Read the model definition and answer for the solid it produces. Units are mm, in the model's axes. Face numbers are marked on the shaded views. A direction names the side the tool comes from. Give positions to 0.01 mm unless a question says otherwise; leave off trailing zeros. Order: outer loops, then holes, each group sorted by start corner. A loop starts at its lowest first (then second) coordinate and runs counter-clockwise, first axis right, second up. Notation, with made-up numbers: (64.25, 17) -> (86.25, 17) arc R13 cw to (86.25, 31) -> close; hole circle Ø9 at (10.25, 18.5). An arc over 180 degrees is marked (long way). Answer as CSV lines item,"result". Start each with the question number.
1) Find section A-A (x = -8.5). Determine the outline of the cut face in (y, z), and give its area (3 significant figures).
2) Find section B-B (z = 61). Determine the outline of the cut face in (x, y).
3) The mould has two halves that part along X. Classify the marked faces 6, 7 and 8: +X half, -X half, draft (parallel to the pull), parting line (faces both ways), or undercut.
4) For the marked faces 1, 2, 3, 4 and 5, determine the directions among +Z, -Z, +X, -X, +Y, -Y from which every point of the face is accessible in a straight line to the end or side of a thin tool.
5) Straight lines are drawn through the part: L1, parallel to Z at x = -5, y = -15.5; L2, parallel to Z at x = -21, y = -19.25; L3, parallel to X at y = -24.75, z = 2. For each, find the intervals that lie inside material, in ascending order. Write a range as from..to.
6) Flat-ended cylindrical pins translate along their axes: pin 1 Ø8 at (x, y) = (19, -19.5) entering from +Z; pin 2 Ø12 at (y, z) = (-16, 94.5) entering from -X; pin 3 Ø1 at (y, z) = (-5, 99) entering from +X. Find the tip coordinate at first contact, or state that the pin passes through.
7) Find section C-C (y = -15). Determine the outline of the cut face in (x, z), and give its area (3 significant figures).
8) Find section D-D (x = -23.5). Determine the outline of the cut face in (y, z).
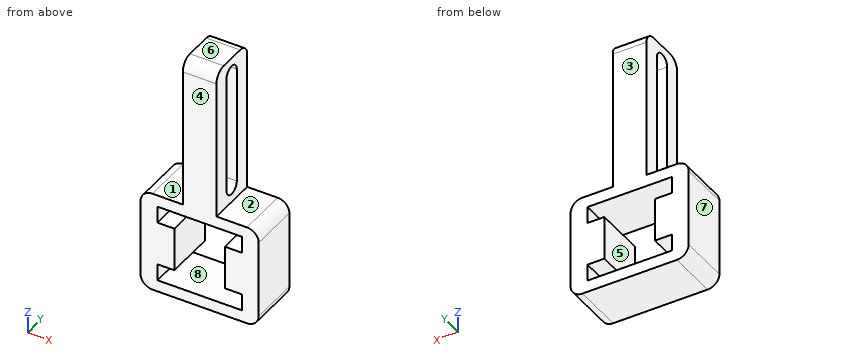
```python
from build123d import *

# Parameters (mm, degrees)
F0_W     = 20
F0_H     = 90
F1_DEPTH = 30
F3_DEPTH = 82
F5_R     = 7
F7_DEPTH = 40.5


with BuildPart() as f1:
    # F0 (on Front) → F1 (new body)
    with BuildSketch(Plane.XZ):
        with BuildLine():
            Line((-28, -30), (28, -30))
            ThreePointArc((28, -30), (32.949747, -27.949747), (35, -23))
            Line((35, -23), (35, 23))
            ThreePointArc((35, 23), (32.949747, 27.949747), (28, 30))
            Line((28, 30), (10, 30))
            Line((10, 30), (-10, 30))
            Line((-10, 30), (-28, 30))
            ThreePointArc((-28, 30), (-32.949747, 27.949747), (-35, 23))
            Line((-35, 23), (-35, -23))
            ThreePointArc((-35, -23), (-32.949747, -27.949747), (-28, -30))
        make_face()
        with Locations((0, 75)):
            Rectangle(F0_W, F0_H)
    extrude(amount=F1_DEPTH)


with BuildPart() as f3:
    # F2 (on face) → F3 (new body, symmetric)
    with BuildSketch(Plane.XZ.offset(30)):
        Polygon((25, 23.023667), (0, 23.023667), (-25, 23.023667), (-25, 13.023667), (-15, 13.023667), (-15, 0.299923), (-15, -0.299923), (-15, -13.023667), (-25, -13.023667), (-25, -23.023667), (0, -23.023667), (25, -23.023667), (25, -13.023667), (15, -13.023667), (15, -0.299923), (15, 0.299923), (15, 13.023667), (25, 13.023667), align=None)
    extrude(amount=F3_DEPTH, both=True)


with BuildPart() as f1_1:
    add(f1.part)

    # F4: cut F3
    add(f3.part, mode=Mode.SUBTRACT)

    # F5
    f5_edges = [f1_1.edges().sort_by_distance(p)[0] for p in [
        (0, -30, 120),
        (0, 0, 120),
    ]]
    fillet(f5_edges, radius=F5_R)


with BuildPart() as f7:
    # F6 (on face) → F7 (new body)
    with BuildSketch(Plane.YZ.offset(10)):
        with BuildLine():
            ThreePointArc((-10.195938, 110), (-15.195938, 115), (-20.195938, 110))
            Line((-20.195938, 110), (-20.195938, 40))
            ThreePointArc((-20.195938, 40), (-15.195938, 35), (-10.195938, 40))
            Line((-10.195938, 40), (-10.195938, 110))
        make_face()
    extrude(amount=-F7_DEPTH)


with BuildPart() as f1_2:
    add(f1_1.part)

    # F8: cut F7
    add(f7.part, mode=Mode.SUBTRACT)


solid = f1_2.part
```
Findings below:
1,outline,"(-30, -30) -> (0, -30) -> (0, -23.02) -> (-30, -23.02) -> close; (-30, 23.02) -> (0, 23.02) -> (0, 113) arc R7 ccw to (-7, 120) -> (-23, 120) arc R7 ccw to (-30, 113) -> close; hole (-20.2, 40) arc R5 ccw to (-10.2, 40) -> (-10.2, 110) arc R5 ccw to (-20.2, 110) -> close"
1,area,"2,320 mm²"
2,outline,"(-10, -30) -> (10, -30) -> (10, -20.2) -> (-10, -20.2) -> close; (-10, -10.2) -> (10, -10.2) -> (10, 0) -> (-10, 0) -> close"
3,face 6,"draft"
3,face 7,"-X half"
3,face 8,"undercut"
4,face 1,"+Z, -X, +Y, -Y"
4,face 2,"+Z, +X, +Y, -Y"
4,face 3,"+Z, -Z, +X, -X, +Y"
4,face 4,"+Z, -Z, +X, -X, -Y"
4,face 5,"+Y, -Y"
5,L1,"-30..-23.02, 23.02..35.01, 114.99..120"
5,L2,"-30..-23.02, -13.02..13.02, 23.02..30"
5,L3,"-35..-15, 15..35"
6,pin 1,"z = 30"
6,pin 2,"x = -10"
6,pin 3,"x = 10"
7,outline,"(-35, -23) arc R7 ccw to (-28, -30) -> (28, -30) arc R7 ccw to (35, -23) -> (35, 23) arc R7 ccw to (28, 30) -> (10, 30) -> (10, 35) -> (-10, 35) -> (-10, 30) -> (-28, 30) arc R7 ccw to (-35, 23) -> close; (-10, 115) -> (10, 115) -> (10, 120) -> (-10, 120) -> close; hole (-25, -23.02) -> (25, -23.02) -> (25, -13.02) -> (15, -13.02) -> (15, 13.02) -> (25, 13.02) -> (25, 23.02) -> (-25, 23.02) -> (-25, 13.02) -> (-15, 13.02) -> (-15, -13.02) -> (-25, -13.02) -> close"
7,area,"2,580 mm²"
8,outline,"(-30, -30) -> (0, -30) -> (0, -23.02) -> (-30, -23.02) -> close; (-30, -13.02) -> (0, -13.02) -> (0, 13.02) -> (-30, 13.02) -> close; (-30, 23.02) -> (0, 23.02) -> (0, 30) -> (-30, 30) -> close"
